Autodesk Inventor part; units mm, degrees
ref_plane "YZ Plane" through (0, 0, 0) normal (1, 0, 0) x (0, 1, 0)
ref_plane "XZ Plane" through (0, 0, 0) normal (0, 1, 0) x (-1, 0, 0)
ref_plane "XY Plane" through (0, 0, 0) normal (0, 0, 1) x (1, 0, 0)
sketch "スケッチ1" plane through (0, 0, 0) normal (0, 1, 0) x (-1, 0, 0)
  circle A0 centre (0, 0) radius 100
  dimension "d0" = 200
extrude "押し出し1" add sketch "スケッチ1" along normal blind 5
sketch "スケッチ12" plane through (0, 5, 0) normal (0, 1, 0) x (1, 0, 0)
  circle A0 centre (0, 0) radius 100
  circle A1 centre (0, 0) radius 3.5
  circle A2 centre (0, 0) radius 5
  circle A3 centre (0, 0) radius 7
  circle A4 centre (0, 7) radius 1
  circle A5 centre (-4.9497, 4.9497) radius 1
  circle A6 centre (-7, 0) radius 1
  circle A7 centre (-4.9497, -4.9497) radius 1
  circle A8 centre (0, -7) radius 1
  circle A9 centre (4.9497, -4.9497) radius 1
  circle A10 centre (7, 0) radius 1
  circle A11 centre (4.9497, 4.9497) radius 1
  dimension "d94" = 14
  dimension "d92" = 7
  dimension "d93" = 10
  dimension "d95" = 2
  dimension "d98" = 360
hole "穴5" at (-7, 5, 0) at (-4.9497, 5, 4.9497) at (0, 5, 7) at (0, 5, -7) at (4.9497, 5, -4.9497) at (7, 5, 0) at (4.9497, 5, 4.9497) at (-4.9497, 5, -4.9497) direction (0, -1, 0) diameter 2 depth 8 tip angle 118
sketch "スケッチ13" plane through (0, 5, 0) normal (0, 1, 0) x (1, 0, 0)
  circle A0 centre (0, 0) radius 100
  circle A1 centre (0, 0) radius 5
  dimension "d107" = 10
extrude "押し出し4" cut sketch "スケッチ13" against normal blind 10 contours A1
sketch "スケッチ14" plane through (0, 5, 0) normal (0, 1, 0) x (1, 0, 0)
  circle A0 centre (0, 0) radius 100
  line L0 (0, 0) -> (0, 55)
  line L1 (0, 55) -> (0, 65)
  line L2 (0, 65) -> (0, 85)
  line L3 (0, 65) -> (30, 65)
  line L4 (0, 65) -> (-30, 65)
  line L5 (-30, 65) -> (30, 65)
  line L6 (30, 65) -> (30, 85)
  line L7 (30, 85) -> (-30, 85)
  line L8 (-30, 85) -> (-30, 65)
  line L9 (0, 0) -> (0, -49.1)
  line L10 (0, -49.1) -> (-14.5, -49.1)
  line L11 (-14.5, -49.1) -> (-14.5, -34.1)
  line L12 (-14.5, -34.1) -> (-24.5, -34.1)
  line L13 (-24.5, -34.1) -> (-34.5, -34.1)
  line L14 (-34.5, -34.1) -> (-44.5, -34.1)
  line L15 (-44.5, -34.1) -> (-54.5, -34.1)
  line L16 (-54.5, -34.1) -> (-64.5, -34.1)
  line L17 (-24.5, -64.1) -> (-34.5, -64.1)
  line L18 (-34.5, -64.1) -> (-44.5, -64.1)
  line L19 (-44.5, -64.1) -> (-54.5, -64.1)
  line L20 (-54.5, -64.1) -> (-64.5, -64.1)
  point P0 (-14.5, -64.1)
  point P1 (-7.25, -49.1)
  dimension "d110" = 55
  dimension "d111" = 10
  dimension "d112" = 20
  dimension "d114" = 30
  dimension "d115" = 30
  dimension "d116" = 49.1
  dimension "d117" = 14.5
  dimension "d118" = 15
  dimension "d119" = 10
  dimension "d120" = 10
  dimension "d121" = 10
  dimension "d122" = 10
  dimension "d123" = 10
hole "穴6" at (-30, 5, -85) at (-30, 5, -65) at (0, 5, -85) at (0, 5, -65) at (30, 5, -65) at (30, 5, -85) at (-64.5, 5, 34.1) at (-54.5, 5, 34.1) at (-44.5, 5, 34.1) at (-34.5, 5, 34.1) at (-24.5, 5, 34.1) at (-14.5, 5, 34.1) at (-64.5, 5, 64.1) at (-54.5, 5, 64.1) at (-44.5, 5, 64.1) at (-34.5, 5, 64.1) at (-24.5, 5, 64.1) at (-14.5, 5, 64.1) at (-30, 5, -85) at (-30, 5, -65) direction (0, -1, 0) diameter 3 depth 8 tip angle 118
properties part number "知能ロボコンターンテーブル.dxf" material "アセタール樹脂、白"
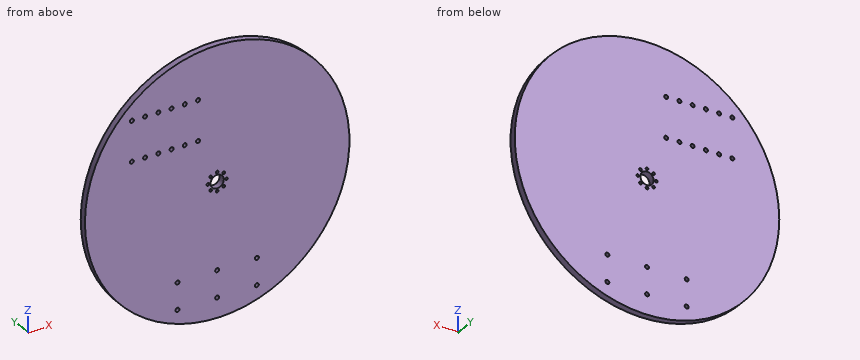
Here's how the part is built. I have some questions about the finished solid (model axes, mm). Round coordinates to 2 decimals unless told otherwise and drop trailing zeros. Loops run counter-clockwise (first coordinate to the right, second up) from the corner with the lowest first, then second, coordinate; pieces in that order, holes last.
1. Suppose I cut it at C-C, the plane z = -79. Please give me the cut outline in (x, y), and give its area (3 significant figures).
Answers:
outline: (-61.31, 0) - (61.31, 0) - (61.31, 5) - (-61.31, 5) - close
area: 613 mm2
2. Will this pin go through, and if not, where does the flat tip stop? pin 1 (1.5 mm diameter, centred on y = 1.5, z = 6.5, fed in from -X).
Answers:
pin 1: stops at x = -99.83
3. Suppose I cut it at A-A, the plane y = 3.3. Give the number of separate pieces and of enclosed holes in the cut face, and give its area (3 significant figures).
Answers:
separate pieces: 1
enclosed holes: 27
area: 31,200 mm2
4. Suppose I cut it at B-B, the plane x = 52.5. Please give me the cut outline in (y, z).
Answers:
outline: (0, -85.11) - (5, -85.11) - (5, 85.11) - (0, 85.11) - close
5. If I drill on probe 1 along Z at (x, y) = (30, 2); probe 2 along Z at (x, y) = (-24.5, 3.25); probe 3 along Z at (x, y) = (-7, 3.2), over which ranges is the centre line in solid material (lowest first)?
Answers:
probe 1: z = -95.39 to -86.5, -83.5 to -66.5, -63.5 to 95.39
probe 2: z = -96.95 to 32.6, 35.6 to 62.6, 65.6 to 96.95
probe 3: z = -99.75 to -1, 1 to 99.75
